Work out the finished part from the listing and answer in its coordinate system (mm). Face numbers are marked on the shaded views. Round coordinates to 2 decimals unless told otherwise and drop trailing zeros. Write each loop counter-clockwise with the first axis right and the second up, starting at its lowest first coordinate (ties: lowest second). Pieces come first, ordered by that corner, then holes.
1. Straight lines are drawn through the part: probe 1 along Y at (x, z) = (-0.65, 0.75); probe 2 along Y at (x, z) = (-0.45, 0.9); probe 3 along X at (y, z) = (-0.25, -0.7). For each, find the intervals that lie inside material, in ascending order.
2. Flat-ended cylindrical pins translate along their axes: pin 1 Ø2 at (x, y) = (0, 0) entering from +Z; pin 2 Ø1 at (x, z) = (1, -0.5) entering from +Y. Find the tip coordinate at first contact, or state that the pin passes through.
3. Find section A-A (z = -0.25). Write down the section's boundary in (x, y), and give its area (3 significant figures).
4. Determine the mould class of the marked faces 1, 2 and 3 for opening direction Y: pulls with the +Y half, pulls with the -Y half, needs draft (parallel to the pull), parting line crosses it, or undercut.
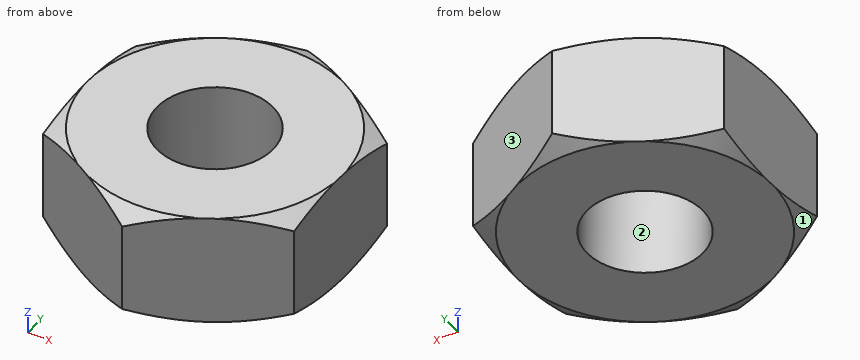
```python
from build123d import *

# Parameters (mm, degrees)
SKETCH2_R           = 1.25
BOSS_EXTRUDE1_DEPTH = 1.2


with BuildPart() as part:
    # Sketch2 → Boss-Extrude1 (new body, symmetric)
    with BuildSketch(Plane.XY):
        Polygon((2.75, 1.58771324), (2.75, -1.58771324), (0, -3.175426481), (-2.75, -1.58771324), (-2.75, 1.58771324), (0, 3.175426481), align=None)
        Circle(SKETCH2_R, mode=Mode.SUBTRACT)
    extrude(amount=BOSS_EXTRUDE1_DEPTH, both=True)

    # Sketch4 → Cut-Revolve2 (revolve, cut)
    with BuildSketch(Plane(origin=(0, 0, 0), x_dir=(0, 0, -1), z_dir=(1, 0, 0))):
        Polygon((1.2, 2.75), (1.2, 4.328660734), (0.2885598, 4.328660734), align=None)
    cut_revolve2 = revolve(axis=Axis((0, 0, 2.99453507), (0, 0, -1)), mode=Mode.SUBTRACT)

    # Mirror1: Cut-Revolve2 across plane
    add(cut_revolve2.mirror(Plane.XY), mode=Mode.SUBTRACT)


solid = part.part
```
Worked answers:
1. probe 1: y = -2.8 to -1.07, 1.07 to 2.8
1. probe 2: y = -2.92 to -1.17, 1.17 to 2.92
1. probe 3: x = -2.75 to -1.22, 1.22 to 2.75
2. pin 1: passes through
2. pin 2: stops at y = 2.89
3. outline: (-2.75, -1.59) - (0, -3.18) - (2.75, -1.59) - (2.75, 1.59) - (0, 3.18) - (-2.75, 1.59) - close; hole circle Ø2.5 at (0, 0)
3. area: 21.3 mm2
4. face 1: pulls with the -Y half
4. face 2: undercut
4. face 3: pulls with the +Y half
